Drawing for the job (mm, zero at the part's lowest x, y, z). A direction names the side the tool comes from. Coordinates: 2 decimals unless noted, no trailing zeros. Order: outer loops, then holes, each group sorted by start corner. A loop starts at its lowest first (then second) coordinate and runs counter-clockwise, first axis right, second up.
1) Wall check: L1, parallel to X at y = 11, z = 15.8; L2, parallel to Y at x = 11, z = 15.75; L3, parallel to Y at x = 35, z = 13. Give the ranges that are in metal, low to high.
2) Tool access for the marked faces 1, 2 and 3: list every direction of +Z, -Z, +X, -X, +Y, -Y with a clear straight run to the whole face (end or side of a thin tool).
3) Cut at B-B (z = 15.5). List the corners of the cut face in (x, y).
4) Pin check, flat tips, straight feed: pin 1 Ø5.5 at (x, z) = (24, 12) entering from -Y; pin 2 Ø3.5 at (y, z) = (5.5, 6) entering from -X; pin 3 Ø7 at (x, y) = (11, 11) entering from -Z. Stop position of each tip, or through.
5) Cut at A-A (x = 29). List the corners of the cut face in (y, z).
6) Cut at C-C (y = 5.5). List the corners of the cut face in (x, z), and give its area (3 significant figures).
7) Mould opens along X. For the marked faces 4, 5 and 6 say: +X half, -X half, draft (parallel to the pull), parting line (faces both ways), or undercut.
8) Cut at D-D (z = 10.25). List the corners of the cut face in (x, y).
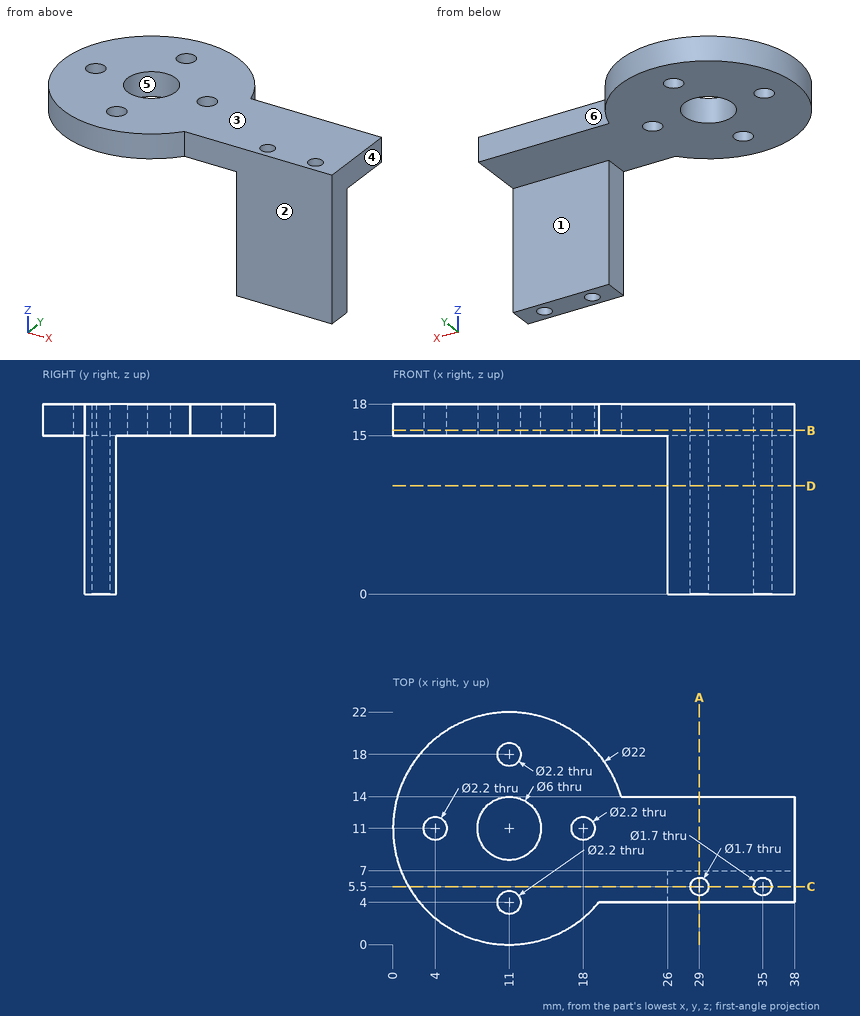
Geometry check:
1. L1: x = 0 to 2.9, 5.1 to 8, 14 to 16.9, 19.1 to 38
1. L2: y = 0 to 2.9, 5.1 to 8, 14 to 16.9, 19.1 to 22
1. L3: y = 4 to 4.65, 6.35 to 7
2. face 1: -Z, +X, -X, +Y
2. face 2: +Z, -Z, +X, -Y
2. face 3: +Z, +X, -X, +Y, -Y
3. outline: (19.49, 4) - (38, 4) - (38, 14) - (21.58, 14) arc R11 ccw (long way) to start; hole circle Ø2.2 at (4, 11); hole circle Ø6 at (11, 11); hole circle Ø2.2 at (11, 4); hole circle Ø2.2 at (11, 18); hole circle Ø2.2 at (18, 11); hole circle Ø1.7 at (29, 5.5); hole circle Ø1.7 at (35, 5.5)
4. pin 1: stops at y = 4
4. pin 2: stops at x = 26
4. pin 3: stops at z = 15
5. outline: (4, 0) - (4.65, 0) - (4.65, 18) - (4, 18) - close; (6.35, 0) - (7, 0) - (7, 15) - (14, 15) - (14, 18) - (6.35, 18) - close
6. outline: (1.47, 15) - (26, 15) - (26, 0) - (28.15, 0) - (28.15, 18) - (1.47, 18) - close; (29.85, 0) - (34.15, 0) - (34.15, 18) - (29.85, 18) - close; (35.85, 0) - (38, 0) - (38, 18) - (35.85, 18) - close
6. area: 228 mm2
7. face 4: +X half
7. face 5: undercut
7. face 6: draft
8. outline: (26, 4) - (38, 4) - (38, 7) - (26, 7) - close; hole circle Ø1.7 at (29, 5.5); hole circle Ø1.7 at (35, 5.5)
